Autodesk Inventor part; units mm, degrees
ref_plane "YZ Plane" through (0, 0, 0) normal (1, 0, 0) x (0, 1, 0)
ref_plane "XZ Plane" through (0, 0, 0) normal (0, 1, 0) x (-1, 0, 0)
ref_plane "XY Plane" through (0, 0, 0) normal (0, 0, 1) x (1, 0, 0)
sketch "Esquisse1" plane through (0, 0, 0) normal (0, 1, 0) x (-1, 0, 0)
  arc A0 (15, 0) -> (-15, 0) centre (0, 0) ccw
  line L0 (-15, 0) -> (15, 0) construction
  line L1 (15, 0) -> (15, -25)
  line L2 (15, -25) -> (-15, -25)
  line L3 (-15, -25) -> (-15, 0)
  arc A1 (-15, 0) -> (15, 0) centre (0, 0) ccw construction
  dimension "d0" = 30
  dimension "d1" = 25
extrude "Extrusion1" add sketch "Esquisse1" along normal blind 15
sketch "Esquisse2" plane through (0, 15, 0) normal (0, 1, 0) x (1, 0, 0)
  arc A0 (-15, 0) -> (15, 0) centre (0, 0) ccw
  circle A1 centre (0, 0) radius 14
  dimension "d4" = 28
extrude "Extrusion2" cut sketch "Esquisse2" against normal blind 13
fillet "Congé1" radius 2 2 edges at (-15, 7.5, -25) (15, 7.5, -25)
properties part number "encoder_shell"
CAD build for the part. Positions are in the model's coordinates, mm. A direction names the side the tool comes from. Give positions to 0.01 mm unless a question says otherwise; leave off trailing zeros. Loops run counter-clockwise (first coordinate to the right, second up) from the corner with the lowest first, then second, coordinate; pieces in that order, holes last. Notation, with made-up numbers: M 14.5,6.5 L 70.5,6.5 A17 cw 70.5,37.5 Z; hole C -7,-18 d11. An arc over 180 degrees is marked long. One line per question, with ' | ' between items. Start each with the question number.
1. Two-plate mould, pull along Z, no slides. Class faces 1 (the face through (0, 0, -5)), 2 (the face through (12.932, 8.591, 5.362)), 3 (the face through (0, 7, -25)): pulls with the +Z half, pulls with the -Z half, needs draft (parallel to the pull), parting line crosses it, or undercut.
2. Saw through at A-A on y = 3.5. Give the cut face in (x, z).
3. Saw through at C-C on x = -12.5. Give the cut face in (y, z), plus the area to 3 significant figures.
4. Probe L1, parallel to X at y = 9, z = 0; L2, parallel to Z at x = 0, y = 5.75; L3, parallel to Y at x = 2.5, z = -8. List the from-to ranges inside material, lowest first. Write a range as from..to.
5. 3-axis set-ups, long thin cutter, end or side, ignore diameter. For faces 4 (the face through (0, 2, 0)), 5 (the face through (0, 7, 15)): which of +Z, -Z, +X, -X, +Y, -Y reach the whole face in a straight line?
6. Saw through at B-B on x = 0. Give the cut face in (y, z).
7. Flat gauge pins, fed straight in: pin 1 (6 mm diameter, centred on x = -3, z = -4, fed in from +Y); pin 2 (4 mm diameter, centred on x = -5, y = 8.5, fed in from +Z); pin 3 (1.5 mm diameter, centred on x = -5.5, y = 9.5, fed in from +Z). Where does each tip first touch, or does it go through?
Result sheet:
1) face 1: needs draft | face 2: undercut | face 3: pulls with the -Z half
2) outline: M -15,-23 A2 ccw -13,-25 L 13,-25 A2 ccw 15,-23 L 15,0 A15 ccw -15,0 Z; hole C 0,0 d28
3) outline: M 0,-25 L 15,-25 L 15,-6.3 L 2,-6.3 L 2,6.3 L 15,6.3 L 15,8.29 L 0,8.29 Z | area: 335 mm^2
4) L1: x = -15..-14, 14..15 | L2: z = -25..-14, 14..15 | L3: y = 0..2
5) face 4: +Y | face 5: +Z, +Y, -Y
6) outline: M 0,-25 L 15,-25 L 15,-14 L 2,-14 L 2,14 L 15,14 L 15,15 L 0,15 Z
7) pin 1: stops at y = 2 | pin 2: stops at z = 14.7 | pin 3: stops at z = 14.23
